Can you work these out from the drawing? Everything is in mm from the part's minimum corner. A direction names the side the tool comes from. Round coordinates to 2 decimals unless told otherwise and drop trailing zeros. Loops run counter-clockwise (first coordinate to the right, second up) from the corner with the lowest first, then second, coordinate; pieces in that order, holes last. Notation, with made-up numbers: (87, 24.25) -> (111, 24.25) arc R24 ccw to (111, 38.25) -> close; hole circle Ø10 at (22.25, 11.5). An arc over 180 degrees is marked (long way). One line per item, written item: value.
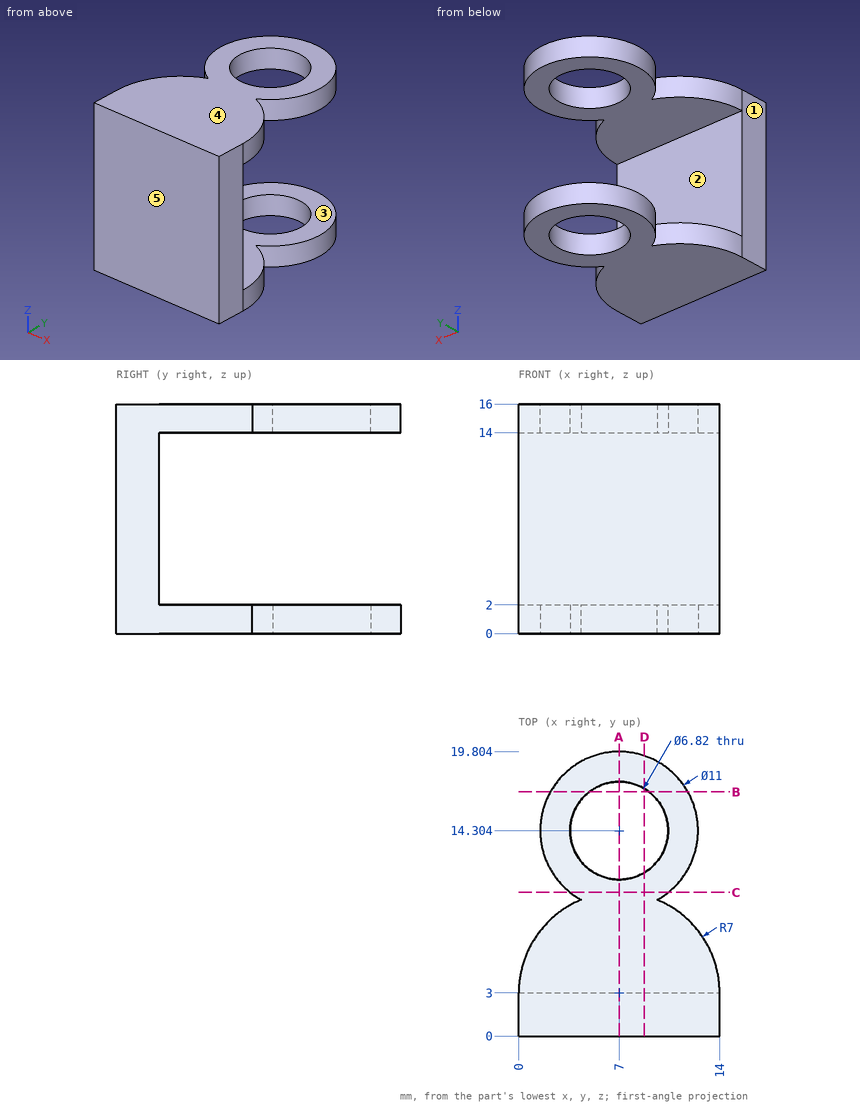
(1) I'm going to push a flat-ended pin straight in: pin 1 Ø6 at (y, z) = (13, 2.5) entering from +X. Where does the tip first touch, or does it pass through?
Recorded:
pin 1: x = 12.5
(2) If we section it at C-C, the plane y = 10: Please give me the cut outline in (x, z), then the cut area to 3 significant figures.
Recorded:
outline: (3.58, 0) -> (10.42, 0) -> (10.42, 2) -> (3.58, 2) -> close; (3.58, 14) -> (10.42, 14) -> (10.42, 16) -> (3.58, 16) -> close
area: 27.4 mm²
(3) If we section it at B-B, the plane y = 17: Please give me the cut outline in (x, z).
Recorded:
outline: (2.21, 0) -> (4.91, 0) -> (4.91, 2) -> (2.21, 2) -> close; (2.21, 14) -> (4.91, 14) -> (4.91, 16) -> (2.21, 16) -> close; (9.09, 0) -> (11.79, 0) -> (11.79, 2) -> (9.09, 2) -> close; (9.09, 14) -> (11.79, 14) -> (11.79, 16) -> (9.09, 16) -> close
(4) If we section it at A-A, the plane x = 7: Please give me the cut outline in (y, z).
Recorded:
outline: (0, 0) -> (10.89, 0) -> (10.89, 2) -> (3, 2) -> (3, 14) -> (10.89, 14) -> (10.89, 16) -> (0, 16) -> close; (17.71, 0) -> (19.8, 0) -> (19.8, 2) -> (17.71, 2) -> close; (17.71, 14) -> (19.8, 14) -> (19.8, 16) -> (17.71, 16) -> close
(5) For the marked faces 1 and 2, which set-ups out of +Z, -Z, +X, -X, +Y, -Y let a thin tool reach every point of the face, with its end or its side?
Recorded:
face 1: +Z, -Z, -X, +Y, -Y
face 2: +X, -X, +Y
(6) Thinking about a two-plate mould opening in Z: for the marked faces 3, 4 and 5, which applies, released by +Z, released by -Z, zero draft, split by the parting line, or undercut?
Recorded:
face 3: undercut
face 4: released by +Z
face 5: zero draft
(7) If I drill on L1, parallel to Y at x = 7, z = 1.35; L2, parallel to Z at x = 7, y = 7; L3, parallel to Y at x = 13.25, z = 4.25, over which ranges is the centre line in solid material (lowest first)?
Recorded:
L1: 0 to 10.89, 17.71 to 19.8
L2: 0 to 2, 14 to 16
L3: 0 to 3
(8) If we section it at D-D, the plane x = 8.75: Please give me the cut outline in (y, z).
Recorded:
outline: (0, 0) -> (11.38, 0) -> (11.38, 2) -> (3, 2) -> (3, 14) -> (11.38, 14) -> (11.38, 16) -> (0, 16) -> close; (17.23, 0) -> (19.52, 0) -> (19.52, 2) -> (17.23, 2) -> close; (17.23, 14) -> (19.52, 14) -> (19.52, 16) -> (17.23, 16) -> close
